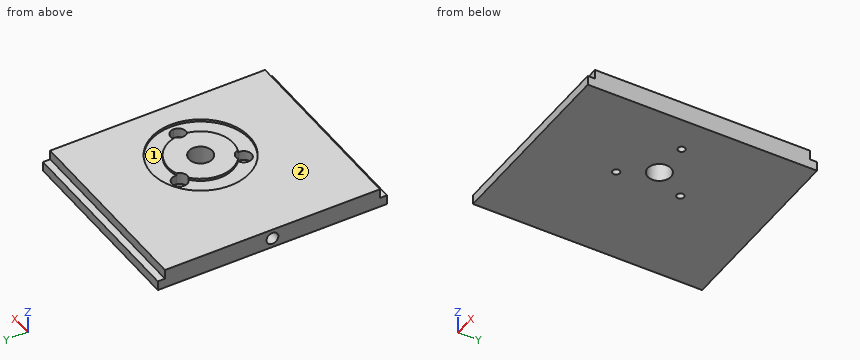
```python
from build123d import *

# Parameters (mm, degrees)
F0_W     = 80
F0_H     = 96
F0_R     = 20.5
F1_DEPTH = 8
F0_R_2   = 4.8708945169
F2_DEPTH = 7
F0_R_3   = 1.5
F3_DEPTH = 3
F4_R     = 2.5
F5_DEPTH = 25
F6_W     = 3
F6_H     = 9.6463483796
F6_H_2   = 12.8309304863
F7_DEPTH = 100


# Not quite as in the source:
# - a feature names something its author has since deleted; it is built from what else it names


with BuildPart() as f1:
    # F0 (on Top) → F1 (new body)
    with BuildSketch(Plane.XY):
        with Locations((-10, 0)):
            Rectangle(F0_W, F0_H)
        Circle(F0_R, mode=Mode.SUBTRACT)
    extrude(amount=F1_DEPTH)



with BuildPart() as f1b:
    # F0 (on Top) → F1, piece 2 (new body)
    with BuildSketch(Plane.XY):
        with BuildLine():
            ThreePointArc((13.4196774194, -2.4969497313), (12.25, 0), (13.4196774194, 2.4969497313))
            ThreePointArc((13.4196774194, 2.4969497313), (6.825, 11.8212467617), (-4.5474168104, 12.8702564214))
            ThreePointArc((-4.5474168104, 12.8702564214), (-6.125, 10.6088111964), (-8.8722606089, 10.3733066901))
            ThreePointArc((-8.8722606089, 10.3733066901), (-13.65, 0), (-8.8722606089, -10.3733066901))
            ThreePointArc((-8.8722606089, -10.3733066901), (-6.125, -10.6088111964), (-4.5474168104, -12.8702564214))
            ThreePointArc((-4.5474168104, -12.8702564214), (6.825, -11.8212467617), (13.4196774194, -2.4969497313))
        make_face()
        Circle(F0_R_2, mode=Mode.SUBTRACT)
    extrude(amount=F1_DEPTH)


with BuildPart() as f1_1:
    add(f1.part)

    add(f1b.part)  # F2 merges F1b
    # F0 (on Top) → F2 (join)
    with BuildSketch(Plane.XY):
        Circle(F0_R)
        with BuildLine():
            ThreePointArc((-4.5474168104, 12.8702564214), (6.825, 11.8212467617), (13.4196774194, 2.4969497313))
            ThreePointArc((13.4196774194, 2.4969497313), (16.8786681277, 2.9430892262), (18.75, 0))
            ThreePointArc((18.75, 0), (16.8786681277, -2.9430892262), (13.4196774194, -2.4969497313))
            ThreePointArc((13.4196774194, -2.4969497313), (6.825, -11.8212467617), (-4.5474168104, -12.8702564214))
            ThreePointArc((-4.5474168104, -12.8702564214), (-4.5118759006, -13.1458107676), (-4.5, -13.4233937587))
            ThreePointArc((-4.5, -13.4233937587), (-9.6094559716, -16.0888999938), (-8.8722606089, -10.3733066901))
            ThreePointArc((-8.8722606089, -10.3733066901), (-13.65, 0), (-8.8722606089, 10.3733066901))
            ThreePointArc((-8.8722606089, 10.3733066901), (-9.6094559716, 16.0888999938), (-4.5, 13.4233937587))
            ThreePointArc((-4.5, 13.4233937587), (-4.5118759006, 13.1458107676), (-4.5474168104, 12.8702564214))
        make_face(mode=Mode.SUBTRACT)
    extrude(amount=F2_DEPTH)

    # F0 (on Top) → F3 (join)
    with BuildSketch(Plane.XY):
        with BuildLine():
            ThreePointArc((-4.5, -13.4233937587), (-4.5118759006, -13.1458107676), (-4.5474168104, -12.8702564214))
            ThreePointArc((-4.5474168104, -12.8702564214), (-6.825, -11.8212467617), (-8.8722606089, -10.3733066901))
            ThreePointArc((-8.8722606089, -10.3733066901), (-9.6094559716, -16.0888999938), (-4.5, -13.4233937587))
        make_face()
        with Locations((-7.75, -13.4233937587)):
            Circle(F0_R_3, mode=Mode.SUBTRACT)
        with BuildLine():
            ThreePointArc((-8.8722606089, -10.3733066901), (-6.825, -11.8212467617), (-4.5474168104, -12.8702564214))
            ThreePointArc((-4.5474168104, -12.8702564214), (-6.125, -10.6088111964), (-8.8722606089, -10.3733066901))
        make_face()
        with BuildLine():
            ThreePointArc((13.4196774194, 2.4969497313), (13.5922973918, 1.2537749451), (13.65, 0))
            ThreePointArc((13.65, 0), (13.5922973918, -1.2537749451), (13.4196774194, -2.4969497313))
            ThreePointArc((13.4196774194, -2.4969497313), (16.8786681277, -2.9430892262), (18.75, 0))
            ThreePointArc((18.75, 0), (16.8786681277, 2.9430892262), (13.4196774194, 2.4969497313))
        make_face()
        with Locations((15.5, 0)):
            Circle(F0_R_3, mode=Mode.SUBTRACT)
        with BuildLine():
            ThreePointArc((13.4196774194, -2.4969497313), (13.5922973918, -1.2537749451), (13.65, 0))
            ThreePointArc((13.65, 0), (13.5922973918, 1.2537749451), (13.4196774194, 2.4969497313))
            ThreePointArc((13.4196774194, 2.4969497313), (12.25, 0), (13.4196774194, -2.4969497313))
        make_face()
        with BuildLine():
            ThreePointArc((-8.8722606089, 10.3733066901), (-6.825, 11.8212467617), (-4.5474168104, 12.8702564214))
            ThreePointArc((-4.5474168104, 12.8702564214), (-4.5118759006, 13.1458107676), (-4.5, 13.4233937587))
            ThreePointArc((-4.5, 13.4233937587), (-9.6094559716, 16.0888999938), (-8.8722606089, 10.3733066901))
        make_face()
        with Locations((-7.75, 13.4233937587)):
            Circle(F0_R_3, mode=Mode.SUBTRACT)
        with BuildLine():
            ThreePointArc((-8.8722606089, 10.3733066901), (-6.125, 10.6088111964), (-4.5474168104, 12.8702564214))
            ThreePointArc((-4.5474168104, 12.8702564214), (-6.825, 11.8212467617), (-8.8722606089, 10.3733066901))
        make_face()
    extrude(amount=F3_DEPTH)

    # F4 (on face) → F5 (cut)
    with BuildSketch(Plane(origin=(-50, 0, 0), x_dir=(0, -1, 0), z_dir=(-1, 0, 0))):
        with Locations((0, 4)):
            Circle(F4_R)
    extrude(amount=-F5_DEPTH, mode=Mode.SUBTRACT)

    # F6 (on face) → F7 (cut)
    with BuildSketch(Plane(origin=(-50, 0, 0), x_dir=(0, -1, 0), z_dir=(-1, 0, 0))):
        with Locations((46.5, 8.8231741898)):
            Rectangle(F6_W, F6_H)
        with Locations((-46.5, 10.4154652432)):
            Rectangle(F6_W, F6_H_2)
    extrude(amount=-F7_DEPTH, mode=Mode.SUBTRACT)


solid = f1_1.part
```
CAD build for the part. Positions are in the model's coordinates, mm. Face numbers are marked on the shaded views. Coordinates: 2 decimals unless noted, no trailing zeros. Order: outer loops, then holes, each group sorted by start corner. A loop starts at its lowest first (then second) coordinate and runs counter-clockwise, first axis right, second up. Notation, with made-up numbers: (89.25, 35.5) - (135.25, 35.5) arc R29 cw to (135.25, 60.5) - close; hole circle Ø1 at (83.5, -33). An arc over 180 degrees is marked (long way). Use a Markdown table: item, result. Add a question column.
(1) Flat gauge pins, fed straight in: pin 1 (1.5 mm diameter, centred on x = -34, z = 5, fed in from +Y); pin 2 (8 mm diameter, centred on x = -1, y = -11, fed in from -Z); pin 3 (3 mm diameter, centred on x = -12.5, y = -14, fed in from +Z); pin 4 (1.5 mm diameter, centred on y = 0.5, z = 5, fed in from -X). Where does each tip first touch, or does it go through?
(2) Saw through at C-C (x = 15.5). Give the cut face in (y, z), then the cut area to 3 significant figures.
(3) Saw through at A-A (x = -37). Give the cut face in (y, z), then the cut area to 3 significant figures.
(4) Drill centre lines: line 1 along Y through (x, z) = (0, 7.35); line 2 along Y through (x, z) = (-7.75, 0.9); line 3 along Y through (x, z) = (-7.75, 5). Where is each one in solid material? Low to high. Write a range as [from, to].
(5) Pull direction Y, two halves, no side cores. Call the marked faces 1 and 2: +Y half, -Y half, draft (parallel to the pull), parting line (faces both ways), or undercut.
(6) Saw through at B-B (x = -7.75). Give the cut face in (y, z).
Solved:
| question | item | result |
|---|---|---|
| 1 | pin 1 | stops at y = 45 |
| 1 | pin 2 | stops at z = 0 |
| 1 | pin 3 | stops at z = 7 |
| 1 | pin 4 | stops at x = -25 |
| 2 | outline | (-48, 0) - (-1.5, 0) - (-1.5, 3) - (-3.25, 3) - (-3.25, 7) - (-13.42, 7) - (-13.42, 8) - (-45, 8) - (-45, 4) - (-48, 4) - close; (1.5, 0) - (48, 0) - (48, 4) - (45, 4) - (45, 8) - (13.42, 8) - (13.42, 7) - (3.25, 7) - (3.25, 3) - (1.5, 3) - close |
| 2 | area | 682 mm² |
| 3 | outline | (-48, 0) - (48, 0) - (48, 4) - (45, 4) - (45, 8) - (-45, 8) - (-45, 4) - (-48, 4) - close; hole circle Ø5 at (0, 4) |
| 3 | area | 724 mm² |
| 4 | line 1 | y = [-45, -20.5], [-13.65, -4.87], [4.87, 13.65], [20.5, 45] |
| 4 | line 2 | y = [-48, -14.92], [-11.92, 11.92], [14.92, 48] |
| 4 | line 3 | y = [-45, -16.67], [-10.17, 10.17], [16.67, 45] |
| 5 | face 1 | undercut |
| 5 | face 2 | draft |
| 6 | outline | (-48, 0) - (-14.92, 0) - (-14.92, 3) - (-16.67, 3) - (-16.67, 7) - (-18.98, 7) - (-18.98, 8) - (-45, 8) - (-45, 4) - (-48, 4) - close; (-11.92, 0) - (11.92, 0) - (11.92, 3) - (10.17, 3) - (10.17, 8) - (-10.17, 8) - (-10.17, 3) - (-11.92, 3) - close; (14.92, 0) - (48, 0) - (48, 4) - (45, 4) - (45, 8) - (18.98, 8) - (18.98, 7) - (16.67, 7) - (16.67, 3) - (14.92, 3) - close |
